```python
from build123d import *

# Parameters (mm, degrees)
SKETCH1_W           = 30
SKETCH1_H           = 20
SKETCH1_R           = 1.5
BOSS_EXTRUDE1_DEPTH = 3
FILLET1_R           = 1


with BuildPart() as part:
    # Sketch1 → Boss-Extrude1 (new body)
    with BuildSketch(Plane(origin=(0, 0, 0), x_dir=(1, 0, 0), z_dir=(0, 1, 0))):
        with Locations((15, 10)):
            Rectangle(SKETCH1_W, SKETCH1_H)
        with Locations((5, 10)):
            Circle(SKETCH1_R, mode=Mode.SUBTRACT)
    extrude(amount=BOSS_EXTRUDE1_DEPTH)

    # Fillet1
    fillet1_edges = [part.edges().sort_by_distance(p)[0] for p in [
        (0, 1.5, -20),
        (30, 1.5, -20),
        (30, 1.5, 0),
        (0, 1.5, 0),
    ]]
    fillet(fillet1_edges, radius=FILLET1_R)


solid = part.part
```
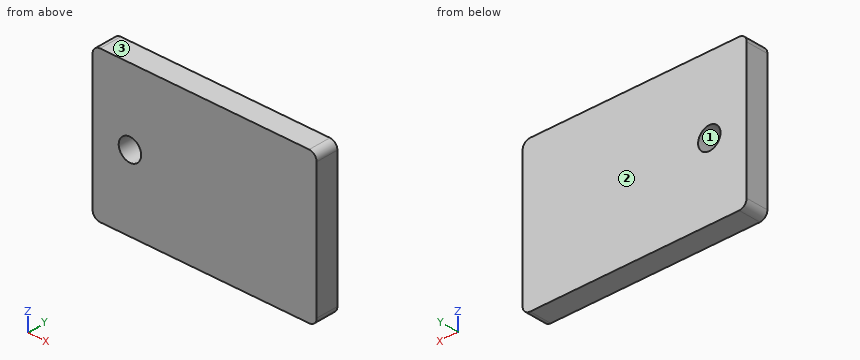
Design review of the part built by this model. Coordinates are the model's own, in mm. Face numbers are marked on the shaded views. Coordinates: 2 decimals unless noted, no trailing zeros. Order: outer loops, then holes, each group sorted by start corner. A loop starts at its lowest first (then second) coordinate and runs counter-clockwise, first axis right, second up. Notation, with made-up numbers: (-33.75, 66.5) -> (-21.75, 66.5) arc R7 cw to (-21.75, 78.5) -> close; hole circle Ø3 at (-38, -16.5). An arc over 180 degrees is marked (long way). One line per item, written item: value. Start each with the question number.
Q1. Insertion check: pin 1 Ø12 at (x, z) = (21.5, -2) entering from -Y. The pin has a flat end and moves straight along its axis. Give the tip position at first contact, or say it passes through.
Q2. Take a section at A-A, the plane z = -10. State the section outline as (x, y) points.
Q3. Mouldability with a two-part tool opening along Z and no side actions: class the marked faces 1, 2 and 3 as pulls with the +Z half, pulls with the -Z half, needs draft (parallel to the pull), parting line crosses it, or undercut.
Q4. For probe 1 along Z at (x, y) = (5, 1.7); probe 2 along X at (y, z) = (0.75, -10), list the stretches that pass through material, from the lowest coordinate up.
Q5. Take a section at B-B, the plane x = 5. State the section outline as (y, z) points, then the cut area to 3 significant figures.
Values follow:
1. pin 1: stops at y = 0
2. outline: (0, 0) -> (3.5, 0) -> (3.5, 3) -> (0, 3) -> close; (6.5, 0) -> (30, 0) -> (30, 3) -> (6.5, 3) -> close
3. face 1: undercut
3. face 2: needs draft
3. face 3: pulls with the +Z half
4. probe 1: z = -20 to -11.5, -8.5 to 0
4. probe 2: x = 0 to 3.5, 6.5 to 30
5. outline: (0, -20) -> (3, -20) -> (3, -11.5) -> (0, -11.5) -> close; (0, -8.5) -> (3, -8.5) -> (3, 0) -> (0, 0) -> close
5. area: 51.0 mm2
